Geometry: final body of the model. Coordinates: model frame, mm. A direction names the side the tool comes from. Round coordinates to 2 decimals unless told otherwise and drop trailing zeros. Write each loop counter-clockwise with the first axis right and the second up, starting at its lowest first coordinate (ties: lowest second). Pieces come first, ordered by that corner, then holes. Notation, with made-up numbers: (81, -7.75) - (116, -7.75) arc R28 cw to (116, 29.25) - close; hole circle Ø2 at (89.5, 88.5). An arc over 180 degrees is marked (long way). Write each question's results on one line, items separated by ' | '.
from build123d import *

# Parameters (mm, degrees)
SKETCH1_W         = 46
SKETCH1_H         = 29.075
EXTRUDE_1_4_DEPTH = 6.2
SKETCH2_R         = 1.75
M4_DRILL_DEPTH    = 6.2
SKETCH3_R         = 1.75
M4_DRILL2_DEPTH   = 8
M4_DRILL3_START   = -8
SKETCH4_R         = 1.75
M4_DRILL3_DEPTH   = 8


with BuildPart() as part:
    # Sketch1 → 1/4 (new body)
    with BuildSketch(Plane.XY):
        Rectangle(SKETCH1_W, SKETCH1_H)
    extrude(amount=EXTRUDE_1_4_DEPTH)

    # Sketch2 → M4_DRILL (cut)
    with BuildSketch(Plane.XY):
        with Locations((-18, 0)):
            Circle(SKETCH2_R)
        with Locations((12, 0)):
            Circle(SKETCH2_R)
    extrude(amount=M4_DRILL_DEPTH, mode=Mode.SUBTRACT)

    # Sketch3 → M4_DRILL2 (cut)
    with BuildSketch(Plane.XZ.offset(14.5375)):
        with Locations(Location((-7, 3.1, 0), (0, 0, 270))):
            Circle(SKETCH3_R)
        with Locations(Location((18, 3.1, 0), (0, 0, 270))):
            Circle(SKETCH3_R)
    extrude(amount=-M4_DRILL2_DEPTH, mode=Mode.SUBTRACT)

    # Sketch4 → M4_DRILL3 (cut)
    with BuildSketch(Plane(origin=(0, 14.5375, 0), x_dir=(1, 0, 0), z_dir=(0, 1, 0)).offset(M4_DRILL3_START)):
        with Locations(Location((18, -3.1, 0), (0, 0, 90))):
            Circle(SKETCH4_R)
        with Locations(Location((-7, -3.1, 0), (0, 0, 90))):
            Circle(SKETCH4_R)
    extrude(amount=M4_DRILL3_DEPTH, mode=Mode.SUBTRACT)


solid = part.part
Q1. Section query C-C, the plane z = 3.1. Return loops of the section in (x, y).
Answer block:
outline: (-23, -14.54) - (-8.75, -14.54) - (-8.75, -6.54) - (-5.25, -6.54) - (-5.25, -14.54) - (16.25, -14.54) - (16.25, -6.54) - (19.75, -6.54) - (19.75, -14.54) - (23, -14.54) - (23, 14.54) - (19.75, 14.54) - (19.75, 6.54) - (16.25, 6.54) - (16.25, 14.54) - (-5.25, 14.54) - (-5.25, 6.54) - (-8.75, 6.54) - (-8.75, 14.54) - (-23, 14.54) - close; hole circle Ø3.5 at (-18, 0); hole circle Ø3.5 at (12, 0)
Q2. Section query B-B, the plane x = -18. Return loops of the section in (y, z), plus the area to 3 significant figures.
Answer block:
outline: (-14.54, 0) - (-1.75, 0) - (-1.75, 6.2) - (-14.54, 6.2) - close; (1.75, 0) - (14.54, 0) - (14.54, 6.2) - (1.75, 6.2) - close | area: 159 mm2
Q3. Mould query, pull axis X, two halves, no side actions, for faces 4 (the flat face through (0, 0, 6.2)), 5 (the flat face through (23, 0, 3)), 6 (the cylindrical face through (-8.55, -10.59, 2.29)). Classes: pulls with the +X half, pulls with the -X half, needs draft (parallel to the pull), parting line crosses it, or undercut.
Answer block:
face 4: needs draft | face 5: pulls with the +X half | face 6: undercut
Q4. Section query D-D, the plane x = -7. Return loops of the section in (y, z).
Answer block:
outline: (-14.54, 0) - (14.54, 0) - (14.54, 1.35) - (6.54, 1.35) - (6.54, 4.85) - (14.54, 4.85) - (14.54, 6.2) - (-14.54, 6.2) - (-14.54, 4.85) - (-6.54, 4.85) - (-6.54, 1.35) - (-14.54, 1.35) - close
Q5. Pin query (flat end, axial travel): pin 1 (3 mm diameter, centred on x = -7, z = 3.1, fed in from -Y); pin 2 (1 mm diameter, centred on x = -7.5, z = 2.5, fed in from +Y). Return the tip coordinate at first contact, or that it passes through.
Answer block:
pin 1: y = -6.54 | pin 2: y = 6.54
Q6. Section query A-A, the plane y = 0. Return loops of the section in (x, z).
Answer block:
outline: (-23, 0) - (-19.75, 0) - (-19.75, 6.2) - (-23, 6.2) - close; (-16.25, 0) - (10.25, 0) - (10.25, 6.2) - (-16.25, 6.2) - close; (13.75, 0) - (23, 0) - (23, 6.2) - (13.75, 6.2) - close
Q7. Access query for faces 1 (the flat face through (18, -6.538, 3)), 2 (the flat face through (18, 6.538, 3)), 3 (the cylindrical face through (-19.75, 0.08, 3.06)). Directions: +Z, -Z, +X, -X, +Y, -Y. A direction counts if a zero-diameter tool reaches every point of the face in a straight line with its end or side. Return the directions, or none.
Answer block:
face 1: -Y | face 2: +Y | face 3: +Z, -Z
Q8. Ray query, line 1 along X through (y, z) = (-8.5, 3.1); line 2 along X through (y, z) = (13, 2); line 3 along Y through (x, z) = (12, 3). Return the intervals inside material, ascending.
Answer block:
line 1: -23 to -8.75, -5.25 to 16.25, 19.75 to 23 | line 2: -23 to -8.36, -5.64 to 16.64, 19.36 to 23 | line 3: -14.54 to -1.75, 1.75 to 14.54
